Source: CAD feature listing. Evaluate the final solid. Frame: model axes, mm. A direction names the side the tool comes from. Give positions to 0.01 mm unless a question says otherwise; leave off trailing zeros. Write each loop counter-clockwise with the first axis right and the second up, starting at its lowest first coordinate (ties: lowest second). Pieces come first, ordered by that corner, then holes. Notation, with made-up numbers: M 5.5,88 L 47.5,88 A21 cw 47.5,107 Z; hole C -39,-8.75 d1. An arc over 180 degrees is marked long. Use CSV: the item, a comma, the result in double quotes. Start each with the question number.
from build123d import *

# Parameters (mm, degrees)
F1_DEPTH = 31.115
F0_R     = 2.350014
F2_DEPTH = 8.89
F3_DEPTH = 19.05


with BuildPart() as f1:
    # F0 (on Top) → F1 (new body)
    with BuildSketch(Plane.XY):
        with BuildLine():
            Line((-32.274887, 32.790409), (-32.274887, 18.16624))
            Line((-32.274887, 18.16624), (-32.274887, -5.944591))
            Line((-32.274887, -5.944591), (-28.24577, -5.944591))
            ThreePointArc((-28.24577, -5.944591), (-22.749887, -9.722416), (-17.254004, -5.944591))
            Line((-17.254004, -5.944591), (-13.224887, -5.944591))
            Line((-13.224887, -5.944591), (-13.224887, 18.16624))
            Line((-13.224887, 18.16624), (-13.224887, 32.790409))
            Line((-13.224887, 32.790409), (-19.685246, 32.790929))
            Line((-19.685246, 32.790929), (-19.685246, 43.633332))
            Line((-19.685246, 43.633332), (-25.806736, 43.633332))
            Line((-25.806736, 43.633332), (-25.806736, 32.790929))
            Line((-25.806736, 32.790929), (-32.274887, 32.790409))
        make_face()
    extrude(amount=F1_DEPTH)

    # F0 (on Top) → F2 (join)
    with BuildSketch(Plane.XY):
        with BuildLine():
            Line((-37.608887, 18.16624), (-37.608887, -11.55176))
            Line((-37.608887, -11.55176), (-7.890887, -11.55176))
            Line((-7.890887, -11.55176), (-7.890887, 18.16624))
            Line((-7.890887, 18.16624), (-13.224887, 18.16624))
            Line((-13.224887, 18.16624), (-13.224887, -5.944591))
            Line((-13.224887, -5.944591), (-17.254004, -5.944591))
            ThreePointArc((-17.254004, -5.944591), (-22.749887, -9.722416), (-28.24577, -5.944591))
            Line((-28.24577, -5.944591), (-32.274887, -5.944591))
            Line((-32.274887, -5.944591), (-32.274887, 18.16624))
            Line((-32.274887, 18.16624), (-37.608887, 18.16624))
        make_face()
        with Locations((-34.560874, -8.21091)):
            Circle(F0_R, mode=Mode.SUBTRACT)
    extrude(amount=F2_DEPTH)

    # F0 (on Top) → F3 (join)
    with BuildSketch(Plane.XY):
        with Locations((-34.560874, -8.21091)):
            Circle(F0_R)
    extrude(amount=F3_DEPTH)


solid = f1.part
1. Section D-D on x = -31. Return loops of the section in (y, z) (3 decimals), then the cut area to 3 significant figures.
2. Section C-C on y = 3.5. Return loops of the section in (x, z) (3 decimals).
3. Pull-direction query (X, two-part tool) for faces 6 (the cylindrical face through (-22.85, -9.72, 19.85)), 7 (the flat face through (-7.891, 3, 4)), 8 (the cylindrical face through (-32.319, -7.505, 13.899)), 9 (the flat face through (-35, -8, 19.05)); classes: released by +X, released by -X, zero draft, split by the parting line, or undercut.
4. Access query for faces 1 (the flat face through (-23, -11.552, 4)), 2 (the flat face through (-15, -5.945, 20)), 3 (the flat face through (-11, 18.166, 4)), 4 (the flat face through (-23, 17, 31.115)), 5 (the flat face through (-35, 18.166, 4)). Directions: +Z, -Z, +X, -X, +Y, -Y. A direction counts if a zero-diameter tool reaches every point of the face in a straight line with its end or side. Return the directions, or none.
5. Section B-B on z = 12. Return loops of the section in (x, y).
6. First-contact query: pin 1 (3 mm diameter, centred on x = -14.5, z = 22.5, fed in from -Y); pin 2 (5 mm diameter, centred on x = -34.5, y = -9, fed in from +Z); pin 3 (1.6 mm diameter, centred on x = -11.5, z = 5, fed in from +Y). Flat tips, straight axial feed; report the tip coordinate or a pass-through.
7. Section A-A on z = 3. Return loops of the section in (x, y).
8. Line query: probe 1 along X at (y, z) = (19, 17); probe 2 along Z at (x, y) = (-11.25, -1); probe 3 along Y at (x, z) = (-31.75, 8). Output: solid intervals per line, ascending.
Resolved:
1,outline,"M -11.552,0 L 32.791,0 L 32.791,31.115 L -5.945,31.115 L -5.945,8.89 L -11.552,8.89 Z"
1,area,"1,260 mm2"
2,outline,"M -37.609,0 L -7.891,0 L -7.891,8.89 L -13.225,8.89 L -13.225,31.115 L -32.275,31.115 L -32.275,8.89 L -37.609,8.89 Z"
3,face 6,"undercut"
3,face 7,"released by +X"
3,face 8,"undercut"
3,face 9,"zero draft"
4,face 1,"+Z, -Z, +X, -X, -Y"
4,face 2,"+Z, +X, -Y"
4,face 3,"+Z, -Z, +X, +Y"
4,face 4,"+Z, +X, -X, +Y, -Y"
4,face 5,"+Z, -Z, -X, +Y"
5,outline,"C -34.56,-8.21 d4.7; M -32.27,-5.94 L -28.25,-5.94 A5.89 ccw -17.25,-5.94 L -13.22,-5.94 L -13.22,32.79 L -19.69,32.79 L -19.69,43.63 L -25.81,43.63 L -25.81,32.79 L -32.27,32.79 Z"
6,pin 1,"stops at y = -5.94"
6,pin 2,"stops at z = 19.05"
6,pin 3,"stops at y = 18.17"
7,outline,"M -37.61,-11.55 L -7.89,-11.55 L -7.89,18.17 L -13.22,18.17 L -13.22,32.79 L -19.69,32.79 L -19.69,43.63 L -25.81,43.63 L -25.81,32.79 L -32.27,32.79 L -32.27,18.17 L -37.61,18.17 Z"
8,probe 1,"x = -32.27 to -13.22"
8,probe 2,"z = 0 to 8.89"
8,probe 3,"y = -11.55 to 32.79"
